from build123d import *

# Parameters (mm, degrees)
SKETCH1_R           = 60
BOSS_EXTRUDE1_DEPTH = 200
SKETCH2_R           = 50
CUT_EXTRUDE1_DEPTH  = 180
FILLET1_R           = 10
SKETCH3_W           = 4.216139726
SKETCH3_H           = 8.515044219
BOSS_EXTRUDE2_DEPTH = 170
SKETCH4_R           = 20
CUT_EXTRUDE3_DEPTH  = 25


with BuildPart() as part:
    # Sketch1 → Boss-Extrude1 (new body)
    with BuildSketch(Plane.XY):
        Circle(SKETCH1_R)
    extrude(amount=BOSS_EXTRUDE1_DEPTH)

    # Sketch2 → Cut-Extrude1 (cut)
    with BuildSketch(Plane.XY.offset(200)):
        Circle(SKETCH2_R)
    extrude(amount=-CUT_EXTRUDE1_DEPTH, mode=Mode.SUBTRACT)

    # Fillet1
    fillet1_edges = [part.edges().sort_by_distance(p)[0] for p in [
        (-60, 0, 0),
    ]]
    fillet(fillet1_edges, radius=FILLET1_R)

    # Sketch3 → Boss-Extrude2 (add)
    with BuildSketch(Plane.XY.offset(20)):
        with Locations((0, 63.882225371)):
            Rectangle(SKETCH3_W, SKETCH3_H)
        Polygon((34.008969531, 49.019783649), (38.612549999, 56.18309468), (35.065707559, 58.462511908), (30.462127092, 51.299200877), align=None)
        Polygon((55.11226167, 22.851429085), (62.857818333, 26.38870629), (61.106370594, 30.223841881), (53.360813931, 26.686564676), align=None)
        Polygon((58.717800132, -10.572092753), (67.146173479, -11.783909894), (67.746192722, -7.610684391), (59.317819375, -6.39886725), align=None)
        Polygon((43.680851933, -40.639049841), (50.116092977, -46.215217947), (52.877077332, -43.028872144), (46.441836288, -37.452704037), align=None)
        Polygon((14.775541879, -57.803395746), (17.174507059, -65.973520844), (21.219863501, -64.785697019), (18.820898322, -56.615571921), align=None)
        Polygon((-18.820898322, -56.615571921), (-21.219863501, -64.785697019), (-17.174507059, -65.973520844), (-14.775541879, -57.803395746), align=None)
        Polygon((-46.441836288, -37.452704037), (-52.877077332, -43.028872144), (-50.116092977, -46.215217947), (-43.680851933, -40.639049841), align=None)
        Polygon((-59.317819375, -6.39886725), (-67.746192722, -7.610684391), (-67.146173479, -11.783909894), (-58.717800132, -10.572092753), align=None)
        Polygon((-53.360813931, 26.686564676), (-61.106370594, 30.223841881), (-62.857818333, 26.38870629), (-55.11226167, 22.851429085), align=None)
        Polygon((-30.462127092, 51.299200877), (-35.065707559, 58.462511908), (-38.612549999, 56.18309468), (-34.008969531, 49.019783649), align=None)
    extrude(amount=BOSS_EXTRUDE2_DEPTH)

    # Sketch4 → Cut-Extrude3 (cut)
    with BuildSketch(Plane(origin=(0, 0, 0), x_dir=(-1, 0, 0), z_dir=(0, 0, -1))):
        Circle(SKETCH4_R)
    extrude(amount=-CUT_EXTRUDE3_DEPTH, mode=Mode.SUBTRACT)


solid = part.part
Read the model definition and answer for the solid it produces. Units are mm, in the model's axes. A direction names the side the tool comes from. Round coordinates to 2 decimals unless told otherwise and drop trailing zeros. Write each loop counter-clockwise with the first axis right and the second up, starting at its lowest first coordinate (ties: lowest second). Pieces come first, ordered by that corner, then holes. Notation, with made-up numbers: M 3,49.5 L 13,49.5 A23 cw 13,63.5 Z; hole C 79,-16.5 d4. An arc over 180 degrees is marked long. Use a Markdown table: item, result.
1) Flat-ended cylindrical pins translate along their axes: pin 1 (2 mm diameter, centred on x = -58, y = 26, fed in from +Z); pin 2 (6 mm diameter, centred on x = -23.5, z = 140, fed in from -Y); pin 3 (3 mm diameter, centred on y = 5.5, z = 97.5, fed in from +X). Find the tip coordinate at first contact, or state that the pin passes through.
Answers follow:
| item | result |
|---|---|
| pin 1 | stops at z = 190 |
| pin 2 | stops at y = -65 |
| pin 3 | stops at x = 59.87 |
2) The part is cut by section A-A (y = 0). Write down the section's boundary in (x, z).
Answers follow:
| item | result |
|---|---|
| outline | M -60,10 A10 ccw -50,0 L -20,0 L -20,20 L -50,20 L -50,200 L -60,200 Z; M 20,0 L 50,0 A10 ccw 60,10 L 60,200 L 50,200 L 50,20 L 20,20 Z |
3) Straight lines are drawn through the part: line 1 along Y through (x, z) = (0, 135.5); line 2 along Z through (x, y) = (-8, 34.5); line 3 along X through (y, z) = (5, 152). For each, find the intervals that lie inside material, in ascending order. Write a range as [from, to].
Answers follow:
| item | result |
|---|---|
| line 1 | y = [-60, -50], [50, 68.14] |
| line 2 | z = [0, 20] |
| line 3 | x = [-59.79, -49.75], [49.75, 59.79] |
4) A tool of negligible diameter and unlimited length cuts with its end or side. For faces 1 (the flat face through (46.98, -43.5, 103.81)), 2 (the flat face through (59.09, 24.67, 103.81)), 3 (the flat face through (-48, -42, 190)), 4 (the flat face through (-32.82, 54.97, 103.81)), 5 (the flat face through (-18, -61, 20)), from which of +Z, -Z, +X, -X, +Y, -Y can it reach the whole face along a straight path? Write none if from no direction.
Answers follow:
| item | result |
|---|---|
| face 1 | +Z, -Z, -Y |
| face 2 | +Z, -Z, +X |
| face 3 | +Z, -X, -Y |
| face 4 | +Z, -Z, +Y |
| face 5 | -Z, -X, -Y |
5) For a pull along X with two mould halves and no side action, classify faces 6 (the flat face through (20.084, -60.918, 103.81)), 7 (the flat face through (-57.335, 28.502, 103.81)), 8 (the flat face through (0, 64, 190)) as pulls with the +X half, pulls with the -X half, needs draft (parallel to the pull), parting line crosses it, or undercut.
Answers follow:
| item | result |
|---|---|
| face 6 | pulls with the +X half |
| face 7 | undercut |
| face 8 | needs draft |
